```python
from build123d import *

# Parameters (mm, degrees)
F1_DEPTH = 15


with BuildPart() as f1:
    # F0 (on Top) → F1 (new body)
    with BuildSketch(Plane.XY):
        Polygon((-5, 0), (0, 0), (0, 5), (-25, 20), (-30, 20), (-30, 15), align=None)
        Polygon((0, 5), (0, 0), (5, 0), (30, 15), (30, 20), (25, 20), align=None)
        Polygon((5, 0), (0, 0), (-5, 0), (-30, 0), (-30, -5), (30, -5), (30, 0), align=None)
    extrude(amount=F1_DEPTH)


solid = f1.part
```
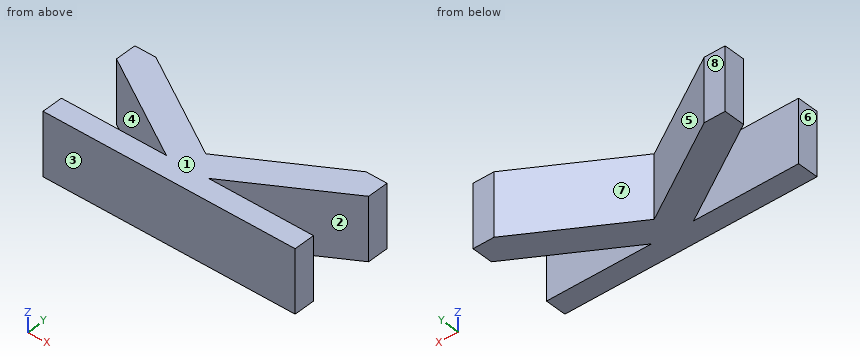
Read the model definition and answer for the solid it produces. Units are mm, in the model's axes. Face numbers are marked on the shaded views. A direction names the side the tool comes from. Coordinates: 2 decimals unless noted, no trailing zeros. Order: outer loops, then holes, each group sorted by start corner. A loop starts at its lowest first (then second) coordinate and runs counter-clockwise, first axis right, second up. Notation, with made-up numbers: (16, -32) - (48, -32) arc R6 cw to (48, -27) - close; hole circle Ø4 at (22.25, 0). An arc over 180 degrees is marked (long way). Answer as a JSON object with one key per item and string values. Group by question number.
Item 1: The mould has two halves that part along X. Classify the marked faces 6, 7 and 8: +X half, -X half, draft (parallel to the pull), parting line (faces both ways), or undercut.
Item 2: Flat-ended cylindrical pins translate along their axes: P1, Ø3, axis at x = 4.5, z = 7, coming from the +Y side; P2, Ø1, axis at x = -8.5, z = 3.5, coming from the +Y side; P3, Ø7.5, axis at x = -18.5, z = 10, coming from the +Y side; P4, Ø8, axis at x = -0.5, y = 14, coming from the -Z side. Find the tip coordinate at first contact, or state that the pin passes through.
Item 3: A tool of negligible diameter and unlimited length cuts with its end or side. For the marked faces 1, 2, 3, 4 and 5, from which of +Z, -Z, +X, -X, +Y, -Y can it reach the whole face along a straight path? Write none if from no direction.
Item 4: Consider probe 1 along X at (y, z) = (12.25, 2.25); probe 2 along Y at (x, z) = (10.5, 5); probe 3 along Y at (x, z) = (-16.5, 8.25). Determine where each line is inside the solid, lowest interval first. Write a range as from..to.
Item 5: Section B-B (y = 17.75) is taken. Give the vertices of the cut face in (x, z).
Item 6: Section C-C (z = 7.5) is taken. Give the vertices of the cut face in (x, y).
Item 7: Section A-A (x = 16.5) is taken. Give the vertices of the cut face in (y, z), plus the area to 3 significant figures.
Results are:
{
 "1": {"face 6": "-X half", "face 7": "undercut", "face 8": "draft"},
 "2": {"P1": "stops at y = 8.6", "P2": "stops at y = 10.4", "P3": "stops at y = 18.35", "P4": "passes through"},
 "3": {"face 1": "+Z, +X, -X, +Y, -Y", "face 2": "+Z, -Z, +X", "face 3": "+Z, -Z, +X, -X, -Y", "face 4": "+Z, -Z, -X", "face 5": "+Z, -Z, +Y"},
 "4": {"probe 1": "x = -25.42..-12.08, 12.08..25.42", "probe 2": "y = -5..0, 3.3..11.3", "probe 3": "y = -5..0, 6.9..14.9"},
 "5": {"outline": "(-30, 0) - (-21.25, 0) - (-21.25, 15) - (-30, 15) - close; (21.25, 0) - (30, 0) - (30, 15) - (21.25, 15) - close"},
 "6": {"outline": "(-30, -5) - (30, -5) - (30, 0) - (5, 0) - (30, 15) - (30, 20) - (25, 20) - (0, 5) - (-25, 20) - (-30, 20) - (-30, 15) - (-5, 0) - (-30, 0) - close"},
 "7": {"outline": "(-5, 0) - (0, 0) - (0, 15) - (-5, 15) - close; (6.9, 0) - (14.9, 0) - (14.9, 15) - (6.9, 15) - close", "area": "195 mm^2"}
}
